Build history of the part. All positions in model axes, mm. Round coordinates to 2 decimals unless told otherwise and drop trailing zeros. Write each loop counter-clockwise with the first axis right and the second up, starting at its lowest first coordinate (ties: lowest second). Pieces come first, ordered by that corner, then holes. Notation, with made-up numbers: M -25.75,-32.5 L -11.75,-32.5 A34 ccw -11.75,-2.5 Z; hole C -12,-16 d6. An arc over 180 degrees is marked long. Use a Markdown table: item, result.
from build123d import *

# Parameters (mm, degrees)
F0_R     = 39.37
F1_DEPTH = 6.35
F2_COUNT = 30


with BuildPart() as f1:
    # F0 (on Top) → F1 (new body)
    with BuildSketch(Plane.XY):
        Circle(F0_R)
        with BuildLine():
            ThreePointArc((-1.9685, -32.9612713309), (-22.6420022304, 24.0345612608), (33.02, 0))
            ThreePointArc((33.02, 0), (24.0353171546, -22.6411998197), (1.9707008312, -32.96113982))
            ThreePointArc((1.9707008312, -32.96113982), (0.0011023785, -33.0199999816), (-1.9685, -32.9612713309))
        make_face(mode=Mode.SUBTRACT)
        with BuildLine():
            ThreePointArc((-0.7022979433, -29.6435257665), (-1.4284612467, -31.2668817673), (-1.9685, -32.9612713309))
            ThreePointArc((-1.9685, -32.9612713309), (0.0011023785, -33.0199999816), (1.9707008312, -32.96113982))
            ThreePointArc((1.9707008312, -32.96113982), (1.4194721848, -31.2703575076), (0.6825926623, -29.6518376845))
            ThreePointArc((0.6825926623, -29.6518376845), (-0.0097619571, -29.6325725152), (-0.7022979433, -29.6435257665))
        make_face()
    extrude(amount=F1_DEPTH)

    # F2: F1 ×30 about axis
    f2_axis = Axis((0, 0, 0), (0, 0, -1))


with BuildPart() as f1_1:
    add(f1.part)
    for i in range(1, F2_COUNT):
        add(f1.part.rotate(f2_axis, i * 360 / F2_COUNT))


solid = f1_1.part
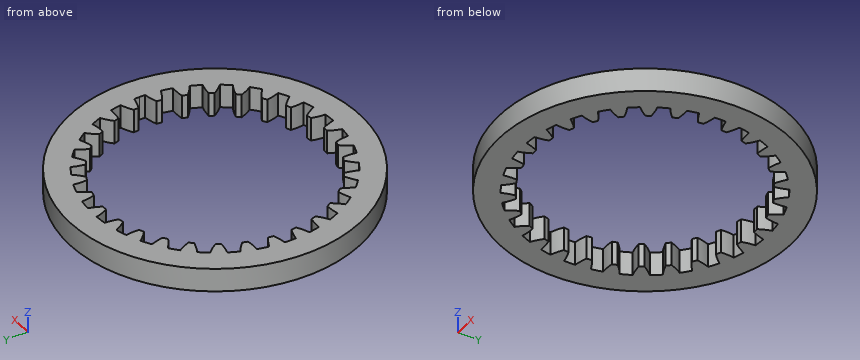
Q1. Cut at A-A on x = 14. Give the cut face in (y, z).
Response values:
| item | result |
|---|---|
| outline | M -36.8,0 L -27.97,0 L -27.97,6.35 L -36.8,6.35 Z; M 27.96,0 L 36.8,0 L 36.8,6.35 L 27.96,6.35 Z |
Q2. Cut at B-B on y = -17. Give the cut face in (x, z).
Response values:
| item | result |
|---|---|
| outline | M -35.51,0 L -26.48,0 L -26.48,6.35 L -35.51,6.35 Z; M 26.47,0 L 35.51,0 L 35.51,6.35 L 26.47,6.35 Z |
Q3. Drill centre lines: L1, parallel to X at y = -0.5, z = 3.25; L2, parallel to X at y = 27, z = 3; L3, parallel to Y at x = -22, z = 2.25. Where is each one in solid material? Low to high.
Response values:
| item | result |
|---|---|
| L1 | x = -39.37 to -33.02, 33.02 to 39.37 |
| L2 | x = -28.65 to -17.48, -12.92 to -12.22, 12.21 to 12.95, 17.49 to 28.65 |
| L3 | y = -32.65 to -24.62, -21.37 to -19.85, 19.85 to 21.41, 24.62 to 32.65 |
Q4. Drop flat-ended pins along their axis: P1, Ø3, axis at x = -24.5, z = 4, coming from the +Y side; P2, Ø3, axis at x = -29, z = 1.5, coming from the +Y side; P3, Ø3, axis at x = -18.5, z = 4, coming from the +Y side. Give the stop position or say it passes through.
Response values:
| item | result |
|---|---|
| P1 | stops at y = 31.95 |
| P2 | stops at y = 28.17 |
| P3 | stops at y = 35.51 |
